Geometry check sheet. Reference: the model listing, model coordinates, mm. Round coordinates to 2 decimals unless told otherwise and drop trailing zeros. Write each loop counter-clockwise with the first axis right and the second up, starting at its lowest first coordinate (ties: lowest second). Pieces come first, ordered by that corner, then holes. Notation, with made-up numbers: (82, 70) -> (100, 70) arc R16 cw to (100, 90) -> close; hole circle Ø2 at (87.5, -27). An arc over 180 degrees is marked (long way). Use a Markdown table: item, result.
```python
from build123d import *

# Parameters (mm, degrees)
SKETCH1_R           = 6
SKETCH1_R_2         = 4.5
BOSS_EXTRUDE1_DEPTH = 600
FILLET3_R           = 1
FILLET4_R           = 1


with BuildPart() as part:
    # Sketch1 → Boss-Extrude1 (new body)
    with BuildSketch(Plane(origin=(0, 0, 0), x_dir=(1, 0, 0), z_dir=(0, 1, 0))):
        Circle(SKETCH1_R)
        Circle(SKETCH1_R_2, mode=Mode.SUBTRACT)
    extrude(amount=BOSS_EXTRUDE1_DEPTH)

    # Fillet3
    fillet3_edges = [part.edges().sort_by_distance(p)[0] for p in [
        (-6, 0, 0),
    ]]
    fillet(fillet3_edges, radius=FILLET3_R)

    # Fillet4
    fillet4_edges = [part.edges().sort_by_distance(p)[0] for p in [
        (-6, 600, 0),
    ]]
    fillet(fillet4_edges, radius=FILLET4_R)


solid = part.part
```
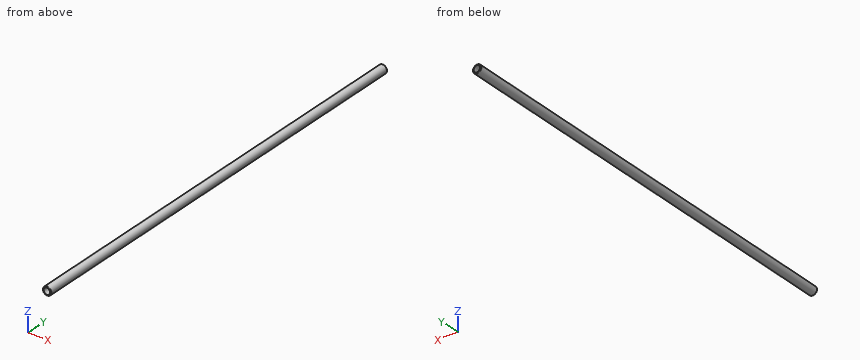
(1) Section check A-A on x = 0. Record the cut outline in (y, z), plus the area to 3 significant figures.
A:
| item | result |
|---|---|
| outline | (0, -5) arc R1 ccw to (1, -6) -> (599, -6) arc R1 ccw to (600, -5) -> (600, -4.5) -> (0, -4.5) -> close; (0, 4.5) -> (600, 4.5) -> (600, 5) arc R1 ccw to (599, 6) -> (1, 6) arc R1 ccw to (0, 5) -> close |
| area | 1,800 mm2 |
(2) Gauge pin test, flat ends, axial feed: pin 1 Ø1.5 at (x, y) = (-3.5, 214) entering from +Z; pin 2 Ø5 at (x, y) = (-1, 321) entering from +Z; pin 3 Ø1.5 at (y, z) = (467, -2.5) entering from +X; pin 4 Ø4 at (x, y) = (-2.5, 403) entering from -Z. Record the tip position at first contact, or that the pin passes through.
A:
| item | result |
|---|---|
| pin 1 | stops at z = 5.33 |
| pin 2 | stops at z = 6 |
| pin 3 | stops at x = 5.74 |
| pin 4 | stops at z = -5.98 |
(3) Section check C-C on y = 532.5. Record the cut outline in (x, z).
A:
| item | result |
|---|---|
| outline | circle Ø12 at (0, 0); hole circle Ø9 at (0, 0) |
(4) Section check B-B on z = 0. Record the cut outline in (x, y), plus the area to 3 significant figures.
A:
| item | result |
|---|---|
| outline | (-6, 1) arc R1 ccw to (-5, 0) -> (-4.5, 0) -> (-4.5, 600) -> (-5, 600) arc R1 ccw to (-6, 599) -> close; (4.5, 0) -> (5, 0) arc R1 ccw to (6, 1) -> (6, 599) arc R1 ccw to (5, 600) -> (4.5, 600) -> close |
| area | 1,800 mm2 |
(5) Thickness scan on line 1 (X direction, y = 271.5, z = 0); line 2 (Z direction, x = 0.75, y = 428). Record the ranges inside material, lowest first.
A:
| item | result |
|---|---|
| line 1 | x = -6 to -4.5, 4.5 to 6 |
| line 2 | z = -5.95 to -4.44, 4.44 to 5.95 |
